```python
from build123d import *

# Parameters (mm, degrees)
BOSS_EXTRUDE1_DEPTH = 4.7625
SKETCH2_R           = 12.7
CUT_EXTRUDE1_DEPTH  = 36.762259699


with BuildPart() as part:
    # Sketch1 → Boss-Extrude1 (new body)
    with BuildSketch(Plane.XY):
        Polygon((2.38125, -25.0625), (15.5375, -25.0625), (15.5375, -20.3), (25.0625, -20.3), (25.0625, 20.3), (20.3, 20.3), (20.3, 25.0625), (-20.3, 25.0625), (-20.3, -15.5375), (-15.5375, -15.5375), (-15.5375, -25.0625), (-2.38125, -25.0625), (-2.38125, -20.3), (2.38125, -20.3), align=None)
    extrude(amount=BOSS_EXTRUDE1_DEPTH)

    # Sketch2 → Cut-Extrude1 (cut, through all)
    with BuildSketch(Plane.XY.offset(4.7625)):
        Circle(SKETCH2_R)
    extrude(amount=-CUT_EXTRUDE1_DEPTH, mode=Mode.SUBTRACT)


solid = part.part
```
Model file for the job. Use its own axes, mm. A direction names the side the tool comes from. Round coordinates to 2 decimals unless told otherwise and drop trailing zeros. Write each loop counter-clockwise with the first axis right and the second up, starting at its lowest first coordinate (ties: lowest second). Pieces come first, ordered by that corner, then holes. Notation, with made-up numbers: (-18, 34.5) -> (7, 34.5) arc R27 ccw to (7, 60.5) -> close; hole circle Ø2 at (18, 9). An arc over 180 degrees is marked (long way). Answer as CSV lines item,"result".
1. Pin check, flat tips, straight feed: pin 1 Ø2.5 at (x, z) = (0.5, 3) entering from -Y; pin 2 Ø2.5 at (x, z) = (24, 3) entering from +Y; pin 3 Ø2.5 at (y, z) = (-18.5, 3) entering from -X. Stop position of each tip, or through.
Resolved:
pin 1,"y = -20.3"
pin 2,"y = 20.3"
pin 3,"x = -15.54"
2. Slice it at D-D, the plane x = 17.5. List the corners of the cut face in (y, z).
Resolved:
outline,"(-20.3, 0) -> (25.06, 0) -> (25.06, 4.76) -> (-20.3, 4.76) -> close"
3. Tool access for faces 5 (the face through (-18, -15.538, 2)), 6 (the face through (15.538, -23, 2)), 7 (the face through (20.3, 23, 2)), 8 (the face through (0, -20.3, 2)): list every direction of +Z, -Z, +X, -X, +Y, -Y with a clear straight run to the whole face (end or side of a thin tool).
Resolved:
face 5,"+Z, -Z, -X, -Y"
face 6,"+Z, -Z, +X, -Y"
face 7,"+Z, -Z, +X, +Y"
face 8,"+Z, -Z, -Y"
4. Mould opens along X. For faces 1 (the face through (2.381, -23, 2)), 2 (the face through (-2.75, -12.4, 2.41)), 3 (the face through (23, 20.3, 2)), 4 (the face through (-15.538, -20, 2)) say: +X half, -X half, draft (parallel to the pull), parting line (faces both ways), or undercut.
Resolved:
face 1,"undercut"
face 2,"undercut"
face 3,"draft"
face 4,"-X half"
5. Drill centre lines: line 1 (Y direction, x = 0, z = 2.2); line 2 (Y direction, x = 17.5, z = 4.6); line 3 (X direction, y = 22, z = 4.25). Where is each one in solid material? Low to high.
Resolved:
line 1,"-20.3 to -12.7, 12.7 to 25.06"
line 2,"-20.3 to 25.06"
line 3,"-20.3 to 20.3"
6. Slice it at C-C, the plane z = 1.8. List the corners of the cut face in (x, y), plus the area to 3 significant figures.
Resolved:
outline,"(-20.3, -15.54) -> (-15.54, -15.54) -> (-15.54, -25.06) -> (-2.38, -25.06) -> (-2.38, -20.3) -> (2.38, -20.3) -> (2.38, -25.06) -> (15.54, -25.06) -> (15.54, -20.3) -> (25.06, -20.3) -> (25.06, 20.3) -> (20.3, 20.3) -> (20.3, 25.06) -> (-20.3, 25.06) -> close; hole circle Ø25.4 at (0, 0)"
area,"1,630 mm²"
7. Slice it at A-A, the plane x = 0. List the corners of the cut face in (y, z).
Resolved:
outline,"(-20.3, 0) -> (-12.7, 0) -> (-12.7, 4.76) -> (-20.3, 4.76) -> close; (12.7, 0) -> (25.06, 0) -> (25.06, 4.76) -> (12.7, 4.76) -> close"
